```python
from build123d import *

# Parameters (mm, degrees)
F2_W     = 2.51875
F2_H     = 14.188414
F2_W_2   = 14.188414
F2_H_2   = 2.51875
F3_DEPTH = 6.35
F4_SIZE  = 1


with BuildPart() as f1:
    # F0 (on Front) → F1 (revolve)
    with BuildSketch(Plane.XZ):
        Polygon((0, 11.25), (0, 0), (38, 0), (38, 4.7625), (15.875, 4.7625), (15.875, 4.76), (6.35, 4.76), (6.35, 11.25), align=None)
    revolve(axis=Axis((19, 0, 0), (1, 0, 0)))

    # F2 (on face) → F3 (cut, through all)
    with BuildSketch(Plane(origin=(0, 0, 0), x_dir=(0, -1, 0), z_dir=(-1, 0, 0))):
        with Locations((-9.990625, 0)):
            Rectangle(F2_W, F2_H)
        with Locations((9.990625, 0)):
            Rectangle(F2_W, F2_H)
        with Locations((0, 9.990625)):
            Rectangle(F2_W_2, F2_H_2)
        with Locations((0, -9.990625)):
            Rectangle(F2_W_2, F2_H_2)
    extrude(amount=-F3_DEPTH, mode=Mode.SUBTRACT)

    # F4
    f4_edges = [f1.edges().sort_by_distance(p)[0] for p in [
        (38, 0, -4.7625),
    ]]
    chamfer(f4_edges, length=F4_SIZE)


solid = f1.part
```
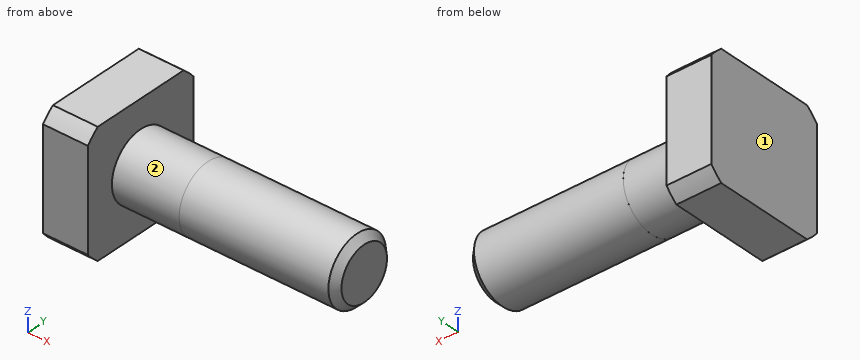
Work out the finished part from the listing and answer in its coordinate system (mm). Face numbers are marked on the shaded views. A direction names the side the tool comes from. Round coordinates to 2 decimals unless told otherwise and drop trailing zeros. Order: outer loops, then holes, each group sorted by start corner. A loop starts at its lowest first (then second) coordinate and runs counter-clockwise, first axis right, second up.
Q1. A cutting plane is placed at D-D, the plane y = -5.75. Determine the outline of the cut face in (x, z).
Solution:
outline: (0, -8.73) - (6.35, -8.73) - (6.35, 8.73) - (0, 8.73) - close
Q2. Find the intervals of material crossed by line 1 along X through (y, z) = (7, 0.5); line 2 along Y through (x, z) = (15, 1); line 3 along Z through (x, y) = (25, 1), in increasing order.
Solution:
line 1: x = 0 to 6.35
line 2: y = -4.65 to 4.65
line 3: z = -4.66 to 4.66
Q3. A tool of negligible diameter and unlimited length cuts with its end or side. For the marked faces 1 and 2, from which of +Z, -Z, +X, -X, +Y, -Y can it reach the whole face along a straight path? Write none if from no direction.
Solution:
face 1: +Z, -Z, -X, +Y, -Y
face 2: +X
Q4. Given pin 1 Ø1.5 at (x, y) = (24, 3.5) entering from +Z; pin 2 Ø2 at (x, y) = (11.5, -6.5) entering from -Z; pin 3 Ø1 at (x, z) = (34, -1) entering from -Y; pin 4 Ø8 at (x, z) = (10.5, -3.5) entering from -Y, each flat-ended and moving along its own axis, determine where each tip first touches the part or whether it passes through.
Solution:
pin 1: stops at z = 3.89
pin 2: passes through
pin 3: stops at y = -4.74
pin 4: stops at y = -4.76
Q5. A cutting plane is placed at C-C, the plane x = 18.5. Determine the outline of the cut face in (y, z) (1 decimal).
Solution:
outline: circle Ø9.5 at (0, 0)
